```python
from build123d import *

# Parameters (mm, degrees)
F1_DEPTH = 25
F2_W     = 8.943856
F2_H     = 1.274483
F3_DEPTH = 25


with BuildPart() as f1:
    # F0 (on Top) → F1 (new body)
    with BuildSketch(Plane.XY):
        Polygon((-4.471928, 3.997871), (0, 3.997871), (-18.293965, 32.363827), (-32.462839, 3.997871), (-27.990839, 3.997871), (-17.725671, 24.548642), align=None)
        Polygon((18.293965, 32.363827), (0, 3.997871), (4.471928, 3.997871), (17.725671, 24.548642), (27.990839, 3.997871), (32.462839, 3.997871), align=None)
    extrude(amount=F1_DEPTH)

    # F2 (on face) → F3 (join)
    with BuildSketch(Plane.XY.offset(25)):
        with Locations((0, 4.635112)):
            Rectangle(F2_W, F2_H)
    extrude(amount=-F3_DEPTH)


solid = f1.part
```
Geometry check sheet. Reference: the model listing, model coordinates, mm. A direction names the side the tool comes from. Give positions to 0.01 mm unless a question says otherwise; leave off trailing zeros. Write each loop counter-clockwise with the first axis right and the second up, starting at its lowest first coordinate (ties: lowest second). Pieces come first, ordered by that corner, then holes. Notation, with made-up numbers: (4, -22) -> (36, -22) arc R32 ccw to (36, 17) -> close; hole circle Ø11 at (74, 37). An arc over 180 degrees is marked (long way). Use one line per item in the form item = value.
Item 1: Access from +Z, -Z, +X, -X, +Y, -Y to the whole of each face (thin tool, end or side, straight path). Record for faces 1 (the flat face through (-5, 11, 25)), 2 (the flat face through (-9.436, 18.628, 12.325)), 3 (the flat face through (11.006, 14.129, 12.325)).
Results list:
face_1 = +Z, +X, -X, +Y, -Y
face_2 = +Z, -Z, +Y
face_3 = +Z, -Z, -Y
Item 2: Depth check by flat-ended pin: pin 1 Ø1 at (x, z) = (12.5, 9) entering from +Y; pin 2 Ø1 at (x, z) = (12, 3) entering from -Y; pin 3 Ø8 at (y, z) = (20.5, 19) entering from -X. Enter the tip coordinate at first touch or a pass-through.
Results list:
pin_1 = 24.16
pin_2 = 14.9
pin_3 = -26.22
Item 3: Scan lines: line 1 (X direction, y = 8.25, z = 5.5); line 2 (X direction, y = 5.75, z = 10.5); line 3 (Y direction, x = 22, z = 5.5). Record each from-to range of solid material in increasing order.
Results list:
line_1 = -30.34 to -25.87, -7.21 to -2.74, 2.74 to 7.21, 25.87 to 30.34
line_2 = -31.59 to -27.12, -5.6 to -1.13, 1.13 to 5.6, 27.12 to 31.59
line_3 = 15.99 to 24.94
Item 4: Sectioned sample at B-B on y = 20.25. Enter the section's corners in (x, z), plus the area to 3 significant figures.
Results list:
outline = (-24.34, 0) -> (-19.87, 0) -> (-19.87, 25) -> (-24.34, 25) -> close; (-14.95, 0) -> (-10.48, 0) -> (-10.48, 25) -> (-14.95, 25) -> close; (10.48, 0) -> (14.95, 0) -> (14.95, 25) -> (10.48, 25) -> close; (19.87, 0) -> (24.34, 0) -> (24.34, 25) -> (19.87, 25) -> close
area = 447 mm2
Item 5: Sectioned sample at C-C on x = -11.5. Enter the section's corners in (y, z).
Results list:
outline = (14.9, 0) -> (21.83, 0) -> (21.83, 25) -> (14.9, 25) -> close
Item 6: Sectioned sample at A-A on z = 13.75. Enter the section's corners in (x, y).
Results list:
outline = (-32.46, 4) -> (-27.99, 4) -> (-17.73, 24.55) -> (-4.47, 4) -> (4.47, 4) -> (17.73, 24.55) -> (27.99, 4) -> (32.46, 4) -> (18.29, 32.36) -> (0.82, 5.27) -> (-0.82, 5.27) -> (-18.29, 32.36) -> close
Item 7: Sectioned sample at D-D on x = -25. Enter the section's corners in (y, z), plus the area to 3 significant figures.
Results list:
outline = (9.99, 0) -> (18.94, 0) -> (18.94, 25) -> (9.99, 25) -> close
area = 224 mm2
Item 8: Mould release check, pull along X, two halves, no side actions. Record for faces 4 (the flat face through (-5, 11, 0)), 5 (the flat face through (22.786, 14.417, 12.325)), 6 (the flat face through (9.68, 19.01, 12.32)), 7 (the flat face through (25.48, 17.98, 12.32)): released by +X, released by -X, zero draft, split by the parting line, or undercut.
Results list:
face_4 = zero draft
face_5 = undercut
face_6 = undercut
face_7 = released by +X
